from build123d import *

# Parameters (mm, degrees)
SKETCH1_W                                   = 160
SKETCH1_H                                   = 160
BOSS_EXTRUDE1_DEPTH                         = 25.4
CBORE_FOR_0_BINDING_HEAD_MACHINE_SC_2_COUNT = 2
CBORE_FOR_0_BINDING_HEAD_MACHINE_SC_2_PITCH = 134.6
CBORE_FOR_0_BINDING_HEAD_MACHINE_SC_3_COUNT = 2
CBORE_FOR_0_BINDING_HEAD_MACHINE_SC_3_PITCH = 190.353145495
CBORE_FOR_0_BINDING_HEAD_MACHINE_SC_4_COUNT = 2
CBORE_FOR_0_BINDING_HEAD_MACHINE_SC_4_PITCH = 134.6
CBORE_FOR_0_BINDING_HEAD_MACHINE_SC_5_COUNT = 2
CBORE_FOR_0_BINDING_HEAD_MACHINE_SC_5_PITCH = 58.400000007
CIRPATTERN1_COUNT                           = 4
SKETCH6_R                                   = 25.4
CUT_EXTRUDE1_DEPTH                          = 26.4


with BuildPart() as part:
    # Sketch1 → Boss-Extrude1 (new body)
    with BuildSketch(Plane(origin=(0, 0, 0), x_dir=(1, 0, 0), z_dir=(0, 1, 0))):
        Rectangle(SKETCH1_W, SKETCH1_H)
    extrude(amount=BOSS_EXTRUDE1_DEPTH)

    # Sketch3 → CBORE for _0 Binding Head Machine Screw1 (revolve, cut)
    with BuildSketch(Plane(origin=(-67.3, 0, -67.3), x_dir=(0, 0, -1), z_dir=(1, 0, 0))):
        Polygon((0, 0), (0, 25.4), (0.80645, 25.4), (0.80645, 0.8128), (1.98501, 0.8128), (1.98501, 0.87249), (2.8575, 0), align=None)
    cbore_for_0_binding_head_machine_screw1 = revolve(axis=Axis((-67.3, -6.35, -67.3), (0, 1, 0)), mode=Mode.SUBTRACT)

    # CBORE for _0 Binding Head Machine Sc 2: CBORE for _0 Binding Head Machine Screw1 ×2
    with Locations(*[(i * CBORE_FOR_0_BINDING_HEAD_MACHINE_SC_2_PITCH, 0, 0) for i in range(1, CBORE_FOR_0_BINDING_HEAD_MACHINE_SC_2_COUNT)]):
        add(cbore_for_0_binding_head_machine_screw1, mode=Mode.SUBTRACT)

    # CBORE for _0 Binding Head Machine Sc 3: CBORE for _0 Binding Head Machine Screw1 ×2
    with Locations(*[Vector(0.707106781, 0, 0.707106781) * (i * CBORE_FOR_0_BINDING_HEAD_MACHINE_SC_3_PITCH) for i in range(1, CBORE_FOR_0_BINDING_HEAD_MACHINE_SC_3_COUNT)]):
        add(cbore_for_0_binding_head_machine_screw1, mode=Mode.SUBTRACT)

    # CBORE for _0 Binding Head Machine Sc 4: CBORE for _0 Binding Head Machine Screw1 ×2
    with Locations(*[(0, 0, i * CBORE_FOR_0_BINDING_HEAD_MACHINE_SC_4_PITCH) for i in range(1, CBORE_FOR_0_BINDING_HEAD_MACHINE_SC_4_COUNT)]):
        add(cbore_for_0_binding_head_machine_screw1, mode=Mode.SUBTRACT)

    # Sketch5 → CBORE for _0 Binding Head Machine Screw2 (revolve, cut)
    with BuildSketch(Plane(origin=(-67.300526968, 25.4, -29.200000004), x_dir=(0, 0, 1), z_dir=(1, 0, 0))):
        Polygon((0, 0), (0, 25.4), (0.80645, 25.4), (0.80645, 0.8128), (1.98501, 0.8128), (1.98501, 0.87249), (2.8575, 0), align=None)
    cbore_for_0_binding_head_machine_screw2 = revolve(axis=Axis((-67.300526968, 31.75, -29.200000004), (0, -1, 0)), mode=Mode.SUBTRACT)

    # CBORE for _0 Binding Head Machine Sc 5: CBORE for _0 Binding Head Machine Screw2 ×2
    with Locations(*[(0, 0, i * CBORE_FOR_0_BINDING_HEAD_MACHINE_SC_5_PITCH) for i in range(1, CBORE_FOR_0_BINDING_HEAD_MACHINE_SC_5_COUNT)]):
        add(cbore_for_0_binding_head_machine_screw2, mode=Mode.SUBTRACT)

    # CirPattern1: CBORE for _0 Binding Head Machine Screw2 ×4 about axis
    cirpattern1_axis = Axis((0, 0, 0), (0, 1, 0))
    for i in range(1, CIRPATTERN1_COUNT):
        add(cbore_for_0_binding_head_machine_screw2.rotate(cirpattern1_axis, i * 360 / CIRPATTERN1_COUNT), mode=Mode.SUBTRACT)

    # CirPattern1 copy 1 sketch → CirPattern1 copy 1 (revolve, cut)
    with BuildSketch(Plane(origin=(29.200000004, 25.4, 67.300526968), x_dir=(1, 0, 0), z_dir=(0, 0, -1))):
        Polygon((0, 0), (0, 25.4), (0.80645, 25.4), (0.80645, 0.8128), (1.98501, 0.8128), (1.98501, 0.87249), (2.8575, 0), align=None)
    revolve(axis=Axis((29.200000004, 31.75, 67.300526968), (0, -1, 0)), mode=Mode.SUBTRACT)

    # CirPattern1 copy 2 sketch → CirPattern1 copy 2 (revolve, cut)
    with BuildSketch(Plane(origin=(67.300526968, 25.4, -29.200000004), x_dir=(0, 0, -1), z_dir=(-1, 0, 0))):
        Polygon((0, 0), (0, 25.4), (0.80645, 25.4), (0.80645, 0.8128), (1.98501, 0.8128), (1.98501, 0.87249), (2.8575, 0), align=None)
    revolve(axis=Axis((67.300526968, 31.75, -29.200000004), (0, -1, 0)), mode=Mode.SUBTRACT)

    # CirPattern1 copy 3 sketch → CirPattern1 copy 3 (revolve, cut)
    with BuildSketch(Plane(origin=(-29.200000004, 25.4, -67.300526968), x_dir=(-1, 0, 0), z_dir=(0, 0, 1))):
        Polygon((0, 0), (0, 25.4), (0.80645, 25.4), (0.80645, 0.8128), (1.98501, 0.8128), (1.98501, 0.87249), (2.8575, 0), align=None)
    revolve(axis=Axis((-29.200000004, 31.75, -67.300526968), (0, -1, 0)), mode=Mode.SUBTRACT)

    # Sketch6 → Cut-Extrude1 (cut, through all)
    with BuildSketch(Plane(origin=(0, 25.4, 0), x_dir=(1, 0, 0), z_dir=(0, 1, 0))):
        Circle(SKETCH6_R)
    extrude(amount=-CUT_EXTRUDE1_DEPTH, mode=Mode.SUBTRACT)


solid = part.part
Here's how the part is built. I have some questions about the finished solid (model axes, mm). A direction names the side the tool comes from. Coordinates: 2 decimals unless noted, no trailing zeros. Loops run counter-clockwise (first coordinate to the right, second up) from the corner with the lowest first, then second, coordinate; pieces in that order, holes last.
1. If we mould it in two halves opening along X, with no side actions, what happens to faces 1 (the flat face through (28, 24.587, 67)), 2 (the flat face through (-1, 13, -80))? For each: pulls with the +X half, pulls with the -X half, needs draft (parallel to the pull), parting line crosses it, or undercut.
2. For P1, Ø3, axis at x = -30, z = 67, coming from the +Y side; P2, Ø4.5, axis at x = -67, z = 67.5, coming from the -Y side; P3, Ø2.5, axis at x = -67.3, z = -29.2, coming from the +Y side, each with a flat end and sliding along its axis, tell me the tip position at first contact or that it passes through.
3. Imagine slicing it at C-C, the plane y = 3. Count the separate pieces of the cut face and the enclosed holes in it, and give its area (3 significant figures).
4. For faces 3 (the flat face through (-67, 0.813, -66)), 4 (the flat face through (-19, 0, -19)), 5 (the flat face through (67, 24.587, -28)), which set-ups out of +Z, -Z, +X, -X, +Y, -Y let a thin tool reach every point of the face, with its end or its side?
5. Imagine slicing it at B-B, the plane z = -14. Please give me the cut outline in (x, y).
6. Imagine slicing it at A-A, the plane x = 0. Please give me the cut outline in (y, z).
7. I need wall thicknesses on L1, parallel to Z at x = 29.2, y = 15.5; L2, parallel to Z at x = -67.3, y = 14.5. Which ranges of each line are inside material? Lowest first, please.
Taken from the geometry:
1. face 1: undercut
1. face 2: needs draft
2. P1: stops at y = 24.9
2. P2: stops at y = 0.25
2. P3: stops at y = 24.59
3. separate pieces: 1
3. enclosed holes: 13
3. area: 23,500 mm2
4. face 3: -Y
4. face 4: +Z, -Z, +X, -X, -Y
4. face 5: +Y
5. outline: (-80, 0) - (-21.19, 0) - (-21.19, 25.4) - (-80, 25.4) - close; (21.19, 0) - (80, 0) - (80, 25.4) - (21.19, 25.4) - close
6. outline: (0, -80) - (25.4, -80) - (25.4, -25.4) - (0, -25.4) - close; (0, 25.4) - (25.4, 25.4) - (25.4, 80) - (0, 80) - close
7. L1: z = -80 to -68.11, -66.49 to 66.49, 68.11 to 80
7. L2: z = -80 to -68.11, -66.49 to -30.01, -28.39 to 28.39, 30.01 to 66.49, 68.11 to 80
